Check sheet for the modelled part. Datum: model origin and axes. Units: mm. Face numbers are marked on the shaded views. A direction names the side the tool comes from. Give positions to 0.01 mm unless a question says otherwise; leave off trailing zeros. Loops run counter-clockwise (first coordinate to the right, second up) from the corner with the lowest first, then second, coordinate; pieces in that order, holes last.
```python
from build123d import *

# Parameters (mm, degrees)
BOSS_EXTRUDE1_DEPTH = 20
SKETCH2_R           = 20
BOSS_EXTRUDE2_DEPTH = 8
CHAMFER1_SIZE       = 0.5
FILLET1_R           = 3


with BuildPart() as part:
    # Sketch1 → Boss-Extrude1 (new body)
    with BuildSketch(Plane.XY):
        with BuildLine():
            Line((0, 69), (0, 82))
            Line((0, 82), (82, 82))
            Line((82, 82), (82, 69))
            ThreePointArc((82, 69), (74, 61), (82, 53))
            Line((82, 53), (82, 29))
            ThreePointArc((82, 29), (74, 21), (82, 13))
            Line((82, 13), (82, 0))
            Line((82, 0), (0, 0))
            Line((0, 0), (0, 13))
            ThreePointArc((0, 13), (8, 21), (0, 29))
            Line((0, 29), (0, 53))
            ThreePointArc((0, 53), (8, 61), (0, 69))
        make_face()
    extrude(amount=BOSS_EXTRUDE1_DEPTH)

    # Sketch2 → Boss-Extrude2 (add)
    with BuildSketch(Plane.XY.offset(20)):
        with Locations((41, 41)):
            Circle(SKETCH2_R)
    extrude(amount=BOSS_EXTRUDE2_DEPTH)

    # Chamfer1
    chamfer1_edges = [part.edges().sort_by_distance(p)[0] for p in [
        (21, 41, 28),
    ]]
    chamfer(chamfer1_edges, length=CHAMFER1_SIZE)

    # Fillet1
    fillet1_edges = [part.edges().sort_by_distance(p)[0] for p in [
        (41, 82, 0),
        (41, 0, 0),
    ]]
    fillet(fillet1_edges, radius=FILLET1_R)


solid = part.part
```
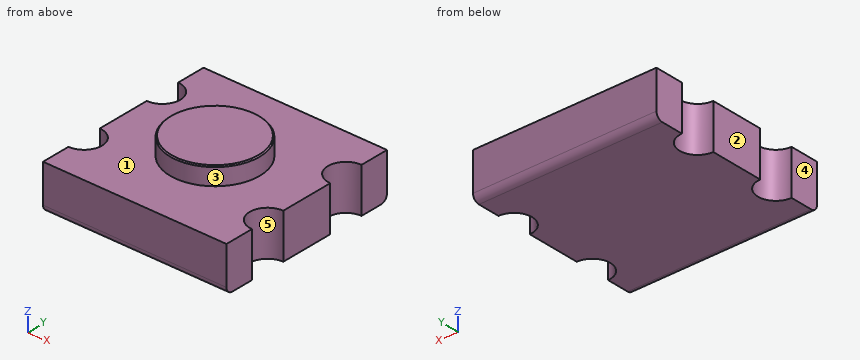
(1) Section check D-D on y = 72. Record the boundary of the cut face in (x, z), plus the area to 3 significant figures.
(2) Section check A-A on y = 41. Record the boundary of the cut face in (x, z), plus the area to 3 significant figures.
(3) Material ranges on line 1 (Y direction, x = 7, z = 1.5); line 2 (Y direction, x = 79, z = 2); line 3 (Z direction, x = 51, y = 19), recorded low to high.
(4) Release check for a two-part mould opening along Y. For the marked faces 3, 4 and 5 record: pulls with the +Y half, pulls with the -Y half, needs draft (parallel to the pull), parting line crosses it, or undercut.
(5) Section check C-C on z = 12.25. Record the boundary of the cut face in (x, y), plus the area to 3 significant figures.
(6) Section check B-B on x = 41. Record the boundary of the cut face in (y, z), plus the area to 3 significant figures.
(7) Access from +Z, -Z, +X, -X, +Y, -Y to the whole of each face (thin tool, end or side, straight path). Record for the marked faces 1 and 2.
Computed values:
1. outline: (0, 0) - (82, 0) - (82, 20) - (0, 20) - close
1. area: 1,640 mm2
2. outline: (0, 0) - (82, 0) - (82, 20) - (61, 20) - (61, 27.5) - (60.5, 28) - (21.5, 28) - (21, 27.5) - (21, 20) - (0, 20) - close
2. area: 1,960 mm2
3. line 1: y = 0.4 to 17.13, 24.87 to 57.13, 64.87 to 81.6
3. line 2: y = 0.17 to 13.58, 28.42 to 53.58, 68.42 to 81.83
3. line 3: z = 0 to 20
4. face 3: parting line crosses it
4. face 4: needs draft
4. face 5: undercut
5. outline: (0, 0) - (82, 0) - (82, 13) arc R8 cw to (82, 29) - (82, 53) arc R8 cw to (82, 69) - (82, 82) - (0, 82) - (0, 69) arc R8 cw to (0, 53) - (0, 29) arc R8 cw to (0, 13) - close
5. area: 6,320 mm2
6. outline: (0, 3) arc R3 ccw to (3, 0) - (79, 0) arc R3 ccw to (82, 3) - (82, 20) - (61, 20) - (61, 27.5) - (60.5, 28) - (21.5, 28) - (21, 27.5) - (21, 20) - (0, 20) - close
6. area: 1,960 mm2
7. face 1: +Z
7. face 2: +Z, -Z, -X, +Y, -Y
